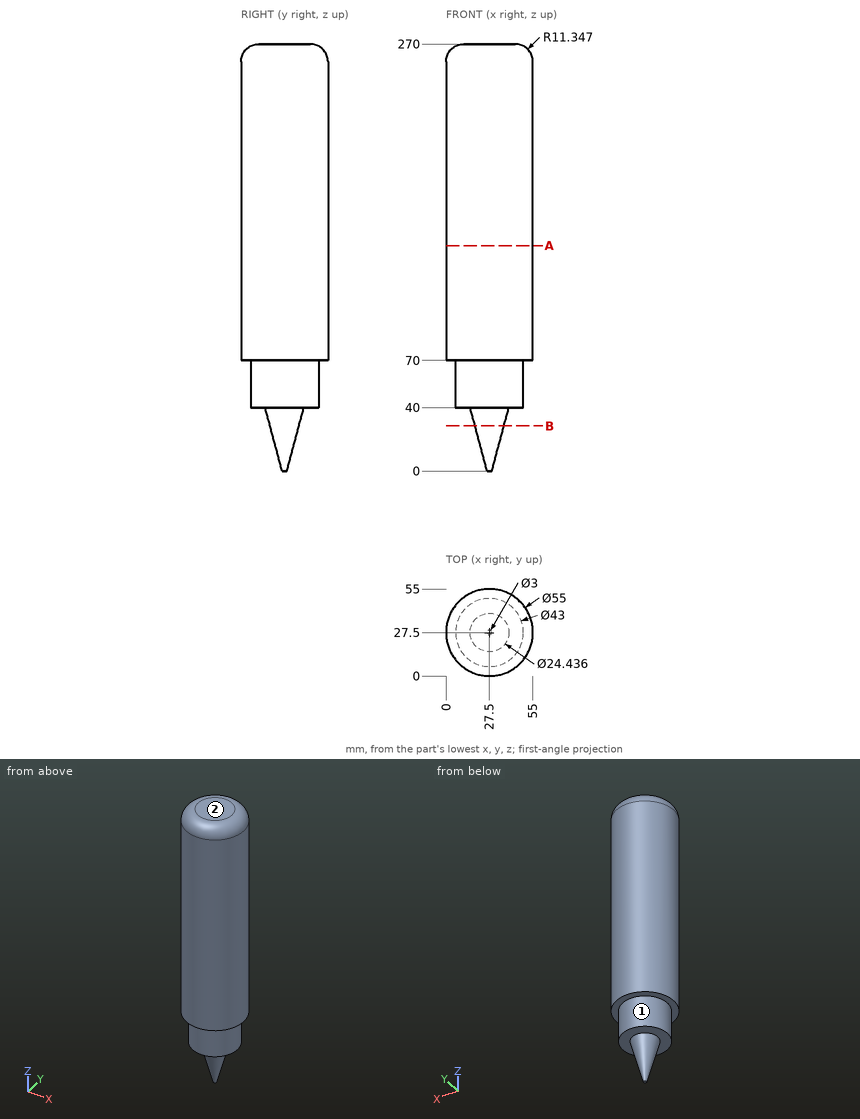
Study the drawing (mm; zero at the part's minimum x, y, z) and answer. A direction names the side the tool comes from. Round coordinates to 2 decimals unless told otherwise and drop trailing zeros. Write each loop counter-clockwise with the first axis right and the second up, starting at its lowest first coordinate (ties: lowest second). Pieces come first, ordered by that corner, then holes. Notation, with made-up numbers: (39.25, -4.75) - (95.25, -4.75) arc R7 ccw to (95.25, 8.25) - close; hole circle Ø8 at (-26, 36). An arc over 180 degrees is marked (long way). Use a Markdown table: item, result. Add a question column.
1. Consider line 1 (Z direction, x = 15, y = 23.5); line 2 (Y direction, x = 26.5, z = 170); line 3 (Z direction, x = 5.5, y = 28) (1 decimal). Determine where each line is inside the solid, lowest interval first.
2. Flat-ended cylindrical pins translate along their axes: P1, Ø1.5, axis at y = 11.5, z = 90, coming from the +X side; P2, Ø2, axis at x = 41, z = 58.5, coming from the +Y side; P3, Ø6, axis at x = 29, z = 214, coming from the -Y side. Find the tip coordinate at first contact, or state that the pin passes through.
3. A tool of negligible diameter and unlimited length cuts with its end or side. For the marked faces 1 and 2, from which of +Z, -Z, +X, -X, +Y, -Y can it reach the whole face along a straight path? Write none if from no direction.
4. The part is cut by section B-B (z = 28.5). Write down the section's boundary in (x, y), and give its area (3 significant figures).
5. The part is cut by section A-A (z = 142.5). Write down the section's boundary in (x, y), and give its area (3 significant figures).
Reported:
| question | item | result |
|---|---|---|
| 1 | line 1 | 40 to 270 |
| 1 | line 2 | 0.02 to 54.98 |
| 1 | line 3 | 70 to 268.4 |
| 2 | P1 | x = 50.38 |
| 2 | P2 | y = 44.99 |
| 2 | P3 | y = 0 |
| 3 | face 1 | -Z |
| 3 | face 2 | +Z, +X, -X, +Y, -Y |
| 4 | outline | circle Ø18.27 at (27.5, 27.5) |
| 4 | area | 262 mm^2 |
| 5 | outline | circle Ø55 at (27.5, 27.5) |
| 5 | area | 2,380 mm^2 |
